from build123d import *

# Parameters (mm, degrees)
BOSS_EXTRUDE1_DEPTH = 2.5
SKETCH3_R           = 18
SKETCH3_R_2         = 10
BOSS_EXTRUDE2_DEPTH = 14


# Read off the part's stored shape, not the designer's step: Dome1
with BuildPart() as part:
    # Sketch1 → Boss-Extrude1 (new body)
    with BuildSketch(Plane(origin=(0, 0, 0), x_dir=(1, 0, 0), z_dir=(0, 1, 0))):
        Polygon((23.094010768, 0), (11.547005384, 20), (-11.547005384, 20), (-23.094010768, 0), (-11.547005384, -20), (11.547005384, -20), align=None)
    extrude(amount=BOSS_EXTRUDE1_DEPTH)

    # Sketch3 → Boss-Extrude2 (add)
    with BuildSketch(Plane.XZ):
        with Locations(Location((0, 0, 0), (0, 0, 90))):
            Circle(SKETCH3_R)
        with Locations(Location((0, 0, 0), (0, 0, 270))):
            Circle(SKETCH3_R_2, mode=Mode.SUBTRACT)
    extrude(amount=BOSS_EXTRUDE2_DEPTH)

    # Dome1 outline → Dome1 (revolve)
    with BuildSketch(Plane.XY):
        with BuildLine():
            Line((0, 2.499999984), (16.000000023, 2.499999984))
            ThreePointArc((16.000000023, 2.499999984), (8.381527321, 6.220887379), (0, 7.5))
            Line((0, 7.5), (0, 2.499999984))
        make_face()
    revolve(axis=Axis((0, 0, 0), (0, 1, 0)))


solid = part.part
Build history of the part. All positions in model axes, mm. A direction names the side the tool comes from. Give positions to 0.01 mm unless a question says otherwise; leave off trailing zeros. Write each loop counter-clockwise with the first axis right and the second up, starting at its lowest first coordinate (ties: lowest second). Pieces come first, ordered by that corner, then holes. Notation, with made-up numbers: (64, 35) - (71, 35) arc R25 ccw to (71, 59) - close; hole circle Ø3 at (83, 15). An arc over 180 degrees is marked (long way). Use one line per item in the form item = value. Start each with the question number.
1. Probe line 1 (X direction, y = -4.75, z = 0); line 2 (Y direction, x = -15, z = -8.5); line 3 (Y direction, x = -7, z = -17.5). List the from-to ranges inside material, lowest first. Write a range as [from, to].
2. Two-plate mould, pull along Z, no slides. Class faces 1 (the face through (14, 0, -12)), 2 (the face through (-9.76, -6.9, 2.17)), 3 (the face through (0, 1, 20)), 4 (the face through (0, 0, 0)): released by +Z, released by -Z, zero draft, split by the parting line, or undercut.
3. Band-saw the part on B-B on z = -15. Write the cut outline in (x, y), plus the area to 3 significant figures.
4. Band-saw the part on C-C on y = -10.5. Write the cut outline in (x, z), plus the area to 3 significant figures.
5. 3-axis set-ups, long thin cutter, end or side, ignore diameter. For faces 5 (the face through (-5.407, -6.902, 17.169)), 6 (the face through (-17.4, 1.23, 9.86)), 7 (the face through (14, 2.5, 9)): which of +Z, -Z, +X, -X, +Y, -Y reach the whole face in a straight line?
6. Band-saw the part on D-D on y = 3.5. Write the cut outline in (x, z), plus the area to 3 significant figures.
7. Drop flat-ended pins along their axis: pin 1 Ø10 at (y, z) = (-10, -4.5) entering from +X; pin 2 Ø1 at (x, y) = (-2, -2.5) entering from -Z; pin 3 Ø4 at (x, z) = (14.5, 0.5) entering from +Y. Give the stop position or say it passes through.
8. Band-saw the part on A-A on x = 0. Write the cut outline in (y, z), plus the area to 3 significant figures.
Conclusion:
q1.line_1 = [-18, -10], [10, 18]
q1.line_2 = [-14, 2.5]
q1.line_3 = [0, 2.5]
q2.face_1 = zero draft
q2.face_2 = undercut
q2.face_3 = released by +Z
q2.face_4 = undercut
q3.outline = (-14.43, 0) - (-9.95, 0) - (-9.95, -14) - (9.95, -14) - (9.95, 0) - (14.43, 0) - (14.43, 2.5) - (5.57, 2.5) arc R23.76 ccw to (-5.57, 2.5) - (-14.43, 2.5) - close
q3.area = 356 mm²
q4.outline = circle Ø36 at (0, 0); hole circle Ø20 at (0, 0)
q4.area = 704 mm²
q5.face_5 = -Y
q5.face_6 = +Z, -X, +Y, -Y
q5.face_7 = +Y
q6.outline = circle Ø28.9 at (0, 0)
q6.area = 656 mm²
q7.pin_1 = 18
q7.pin_2 = -17.94
q7.pin_3 = 4.56
q8.outline = (-14, -18) - (0, -18) - (0, -20) - (2.5, -20) - (2.5, -16) arc R28.1 ccw to (2.5, 16) - (2.5, 20) - (0, 20) - (0, 18) - (-14, 18) - (-14, 10) - (0, 10) - (0, -10) - (-14, -10) - close
q8.area = 433 mm²
